Design review of the part built by this model. Coordinates are the model's own, in mm. A direction names the side the tool comes from. Round coordinates to 2 decimals unless told otherwise and drop trailing zeros. Loops run counter-clockwise (first coordinate to the right, second up) from the corner with the lowest first, then second, coordinate; pieces in that order, holes last. Notation, with made-up numbers: M 72,-38 L 111,-38 A28 ccw 111,-9 Z; hole C 50,-1.75 d5. An arc over 180 degrees is marked long. Use a Markdown table: item, result.
from build123d import *

# Parameters (mm, degrees)
SKETCH1_W           = 15
SKETCH1_H           = 18
BOSS_EXTRUDE1_DEPTH = 1.2
SKETCH2_W           = 3.5
SKETCH2_H           = 6
BOSS_EXTRUDE2_DEPTH = 1
SKETCH3_R           = 0.491511221
CUT_EXTRUDE1_DEPTH  = 1


with BuildPart() as part:
    # Sketch1 → Boss-Extrude1 (new body)
    with BuildSketch(Plane.XY):
        Rectangle(SKETCH1_W, SKETCH1_H)
    extrude(amount=BOSS_EXTRUDE1_DEPTH)

    # Sketch2 → Boss-Extrude2 (add)
    with BuildSketch(Plane.XY.offset(1.2)):
        with Locations((0, -6)):
            Rectangle(SKETCH2_W, SKETCH2_H)
    extrude(amount=BOSS_EXTRUDE2_DEPTH)

    # Sketch3 → Cut-Extrude1 (cut)
    with BuildSketch(Plane.XY.offset(1.2)):
        with Locations((-6.181907245, 8.041418738)):
            Circle(SKETCH3_R)
        with Locations((-4.681907245, 8.041418738)):
            Circle(SKETCH3_R)
        with Locations((-3.181907245, 8.041418738)):
            Circle(SKETCH3_R)
        with Locations((-1.681907245, 8.041418738)):
            Circle(SKETCH3_R)
        with Locations((-0.181907245, 8.041418738)):
            Circle(SKETCH3_R)
        with Locations((1.318092755, 8.041418738)):
            Circle(SKETCH3_R)
        with Locations((2.818092755, 8.041418738)):
            Circle(SKETCH3_R)
        with Locations((4.318092755, 8.041418738)):
            Circle(SKETCH3_R)
        with Locations((5.818092755, 8.041418738)):
            Circle(SKETCH3_R)
    extrude(amount=-CUT_EXTRUDE1_DEPTH, mode=Mode.SUBTRACT)


solid = part.part
1. Take a section at C-C on z = 0.85. Count the separate pieces of the cut face and the enclosed holes in it, and give its area (3 significant figures).
Check values:
| item | result |
|---|---|
| separate pieces | 1 |
| enclosed holes | 9 |
| area | 263 mm² |
2. Insertion check: pin 1 (0.5 mm diameter, centred on x = -5, y = 8, fed in from +Z); pin 2 (1.1 mm diameter, centred on x = -0.5, z = 2, fed in from +Y). Each pin has a flat end and moves straight along its axis. Give the tip position at first contact, or say it passes through.
Check values:
| item | result |
|---|---|
| pin 1 | stops at z = 1.2 |
| pin 2 | stops at y = -3 |
3. Take a section at B-B on x = 0. Give the boundary of the cut face in (y, z).
Check values:
| item | result |
|---|---|
| outline | M -9,0 L 9,0 L 9,1.2 L 8.5,1.2 L 8.5,0.2 L 7.58,0.2 L 7.58,1.2 L -3,1.2 L -3,2.2 L -9,2.2 Z |
4. The part is to be moulded in two halves that separate along X. For faces 1 (the face through (0, 0, 1.2)), 2 (the face through (1.75, -6, 2)), 3 (the face through (4, 8, 0.2)), say which applies: pulls with the +X half, pulls with the -X half, needs draft (parallel to the pull), parting line crosses it, or undercut.
Check values:
| item | result |
|---|---|
| face 1 | needs draft |
| face 2 | pulls with the +X half |
| face 3 | undercut |
5. Machinability: for faces 4 (the face through (0, -9, 1)), 5 (the face through (-0.29, 7.56, 0.71)), which of the approach directions +Z, -Z, +X, -X, +Y, -Y give a long, thin tool a straight path to every point of the face, cutting with its end or side? Answer none if there is none.
Check values:
| item | result |
|---|---|
| face 4 | +Z, -Z, +X, -X, -Y |
| face 5 | +Z |
6. Take a section at D-D on z = 1.95. Give the boundary of the cut face in (x, y).
Check values:
| item | result |
|---|---|
| outline | M -1.75,-9 L 1.75,-9 L 1.75,-3 L -1.75,-3 Z |
7. Wall thickness on line 1 along Y through (x, z) = (-4.75, 0.6); line 2 along Z through (x, y) = (6.5, -7); line 3 along Y through (x, z) = (4, 0.35): over which ranges is each line inside the solid? List them lowest first. Write a range as from..to.
Check values:
| item | result |
|---|---|
| line 1 | y = -9..7.55, 8.53..9 |
| line 2 | z = 0..1.2 |
| line 3 | y = -9..7.67, 8.42..9 |
8. Take a section at A-A on y = -8. Give the boundary of the cut face in (x, z), and give its area (3 significant figures).
Check values:
| item | result |
|---|---|
| outline | M -7.5,0 L 7.5,0 L 7.5,1.2 L 1.75,1.2 L 1.75,2.2 L -1.75,2.2 L -1.75,1.2 L -7.5,1.2 Z |
| area | 21.5 mm² |
